Design review of the part built by this model. Coordinates are the model's own, in mm. A direction names the side the tool comes from. Coordinates: 2 decimals unless noted, no trailing zeros. Write each loop counter-clockwise with the first axis right and the second up, starting at its lowest first coordinate (ties: lowest second). Pieces come first, ordered by that corner, then holes. Notation, with made-up numbers: (28, 19) - (48, 19) arc R7 ccw to (48, 23) - close; hole circle Ø4 at (-8.5, 19.25). An arc over 180 degrees is marked (long way). Answer as a JSON object with one key per item and string values.
```python
from build123d import *

# Parameters (mm, degrees)
BOSS_EXTRUDE1_DEPTH = 4.8
FILLET1_R           = 2.5


with BuildPart() as part:
    # Sketch1 → Boss-Extrude1 (new body)
    with BuildSketch(Plane(origin=(0, 0, 0), x_dir=(0, 1, 0), z_dir=(0, 0, 1))):
        Polygon((-15, -4.9), (-15, -9.9), (-19.8, -9.9), (-19.8, 9.9), (-15, 9.9), (-15, 4.9), (5.2, 4.9), (5.2, 9.9), (10, 9.9), (10, -9.9), (5.2, -9.9), (5.2, -4.9), align=None)
    extrude(amount=BOSS_EXTRUDE1_DEPTH)

    # Fillet1
    fillet1_edges = [part.edges().sort_by_distance(p)[0] for p in [
        (0, -19.8, 4.8),
        (-9.9, -17.4, 4.8),
        (9.9, 10, 2.4),
        (-9.9, 10, 2.4),
        (-9.9, -19.8, 2.4),
        (9.9, -19.8, 2.4),
        (-9.9, 7.6, 4.8),
        (0, 10, 4.8),
        (9.9, 7.6, 4.8),
        (9.9, -17.4, 4.8),
    ]]
    fillet(fillet1_edges, radius=FILLET1_R)


solid = part.part
```
(1) Take a section at D-D, the plane y = -16.5. Write out the cut boundary in (x, z), and give its area (3 significant figures).
Solved:
{"outline": "(-9.9, 0) - (9.9, 0) - (9.9, 2.3) arc R2.5 ccw to (7.4, 4.8) - (-7.4, 4.8) arc R2.5 ccw to (-9.9, 2.3) - close", "area": "92.4 mm^2"}
(2) For pin 1 (1.5 mm diameter, centred on y = -7.5, z = 0.5, fed in from -X); pin 2 (1.5 mm diameter, centred on x = 3, z = 3.5, fed in from +Y); pin 3 (1.4 mm diameter, centred on x = 7, z = 3.5, fed in from +Y), all flat-tipped, find the tip position at first contact; note any pin that passes through.
Solved:
{"pin 1": "stops at x = -4.9", "pin 2": "stops at y = 9.96", "pin 3": "stops at y = 9.95"}
(3) Take a section at B-B, the plane z = 1.3. Write out the cut boundary in (x, y), and give its area (3 significant figures).
Solved:
{"outline": "(-9.9, -17.3) arc R2.5 ccw to (-7.4, -19.8) - (7.4, -19.8) arc R2.5 ccw to (9.9, -17.3) - (9.9, -15) - (4.9, -15) - (4.9, 5.2) - (9.9, 5.2) - (9.9, 7.5) arc R2.5 ccw to (7.4, 10) - (-7.4, 10) arc R2.5 ccw to (-9.9, 7.5) - (-9.9, 5.2) - (-4.9, 5.2) - (-4.9, -15) - (-9.9, -15) - close", "area": "383 mm^2"}
(4) The part is to be moulded in two halves that separate along Y. For faces 4 (the face through (7, -15, 2)), 5 (the face through (0, -5, 0)), 6 (the face through (-9.148, -19.087, 1.166)), 7 (the face through (-4.9, -5, 2)), say which applies: pulls with the +Y half, pulls with the -Y half, needs draft (parallel to the pull), parting line crosses it, or undercut.
Solved:
{"face 4": "undercut", "face 5": "needs draft", "face 6": "pulls with the -Y half", "face 7": "undercut"}
(5) Take a section at A-A, the plane x = -6.75. Write out the cut boundary in (y, z), and give its area (3 significant figures).
Solved:
{"outline": "(-19.8, 0) - (-15, 0) - (-15, 4.8) - (-17.3, 4.8) arc R2.5 ccw to (-19.8, 2.3) - close; (5.2, 0) - (10, 0) - (10, 2.3) arc R2.5 ccw to (7.5, 4.8) - (5.2, 4.8) - close", "area": "43.4 mm^2"}
(6) Take a section at C-C, the plane x = 1.25. Write out the cut boundary in (y, z), and give its area (3 significant figures).
Solved:
{"outline": "(-19.8, 0) - (10, 0) - (10, 2.3) arc R2.5 ccw to (7.5, 4.8) - (-17.3, 4.8) arc R2.5 ccw to (-19.8, 2.3) - close", "area": "140 mm^2"}
(7) Tool access review of faces 1 (the face through (7, 5.2, 2)), 2 (the face through (-9.187, 6.366, 4.048)), 3 (the face through (-7, -15, 2)): name each direction out of +Z, -Z, +X, -X, +Y, -Y from which nothing blocks a thin tool from reaching the whole face with its end or side.
Solved:
{"face 1": "+Z, -Z, +X", "face 2": "+Z, -X, +Y, -Y", "face 3": "+Z, -Z, -X"}
(8) To check wall thickness, follow line 1 (Y direction, x = 6.25, z = 1.55); line 2 (X direction, y = -9, z = 1.4); line 3 (Y direction, x = 5.75, z = 4.6). State the ranges of each line that lie inside material, in increasing order. Write a range as from..to.
Solved:
{"line 1": "y = -19.8..-15, 5.2..10", "line 2": "x = -4.9..4.9", "line 3": "y = -18.28..-15, 5.2..8.48"}
